Can you work these out from the model? Positions are in its coordinate system, mm. A direction names the side the tool comes from. Round coordinates to 2 decimals unless told otherwise and drop trailing zeros. Order: outer loops, then holes, each group sorted by start corner. A loop starts at its lowest first (then second) coordinate and runs counter-clockwise, first axis right, second up. Notation, with made-up numbers: M 80,-19.5 L 122,-19.5 A23 ccw 122,-10.5 Z; hole C 49.5,33.25 d8. An arc over 180 degrees is marked long. One line per question, with ' | ' between items.
```python
from build123d import *

# Parameters (mm, degrees)
SKETCH_1_W          = 40
SKETCH_1_H          = 40
EXTRUDE_1_DEPTH     = 40
SKETCH_2_R          = 10
CUT_EXTRUDE_1_DEPTH = 41
SKETCH_3_W          = 30
SKETCH_3_H          = 20
CUT_EXTRUDE_2_DEPTH = 20
CUT_EXTRUDE_3_DEPTH = 41
CUT_EXTRUDE_4_DEPTH = 41
SKETCH_7_W          = 10
SKETCH_7_H          = 10
CUT_EXTRUDE_5_DEPTH = 20
CUT_EXTRUDE_6_DEPTH = 21


with BuildPart() as part:
    # 草圖1 → 填料-伸長1 (new body)
    with BuildSketch(Plane(origin=(0, 0, 0), x_dir=(1, 0, 0), z_dir=(0, 1, 0))):
        Rectangle(SKETCH_1_W, SKETCH_1_H)
    extrude(amount=EXTRUDE_1_DEPTH)

    # 草圖2 → 除料-伸長1 (cut, through all)
    with BuildSketch(Plane(origin=(0, 40, 0), x_dir=(1, 0, 0), z_dir=(0, 1, 0))):
        Circle(SKETCH_2_R)
        with BuildLine():
            Line((0, -20), (20, -20))
            Line((20, -20), (20, 0))
            ThreePointArc((20, 0), (14.142135624, -14.142135624), (0, -20))
        make_face()
    extrude(amount=-CUT_EXTRUDE_1_DEPTH, mode=Mode.SUBTRACT)

    # 草圖3 → 除料-伸長2 (cut)
    with BuildSketch(Plane(origin=(20, 0, 0), x_dir=(0, 0, -1), z_dir=(1, 0, 0))):
        with Locations((-5, 30)):
            Rectangle(SKETCH_3_W, SKETCH_3_H)
    extrude(amount=-CUT_EXTRUDE_2_DEPTH, mode=Mode.SUBTRACT)

    # 草圖4 → 除料-伸長3 (cut, through all)
    with BuildSketch(Plane.XY.offset(20)):
        Polygon((20, 30), (10, 30), (10, 20), (0, 20), (0, 30), (-10, 40), (20, 40), align=None)
    extrude(amount=-CUT_EXTRUDE_3_DEPTH, mode=Mode.SUBTRACT)

    # 草圖5 → 除料-伸長4 (cut, through all)
    with BuildSketch(Plane(origin=(20, 0, 0), x_dir=(0, 0, -1), z_dir=(1, 0, 0))):
        Polygon((10, 40), (0, 30), (-10, 30), (-20, 20), (-20, 40), align=None)
    extrude(amount=-CUT_EXTRUDE_4_DEPTH, mode=Mode.SUBTRACT)

    # 草圖7 → 除料-伸長5 (cut)
    with BuildSketch(Plane.XY.offset(20)):
        with Locations((-5, 25)):
            Rectangle(SKETCH_7_W, SKETCH_7_H)
    extrude(amount=-CUT_EXTRUDE_5_DEPTH, mode=Mode.SUBTRACT)

    # 草圖9 → 除料-伸長6 (cut, through all)
    with BuildSketch(Plane(origin=(0, 20, 0), x_dir=(1, 0, 0), z_dir=(0, 1, 0))):
        with BuildLine():
            ThreePointArc((-7.071067812, 7.071067812), (-9.238795325, 3.826834324), (-10, 0))
            Line((-10, 0), (-10, 10))
            Line((-10, 10), (0, 10))
            ThreePointArc((0, 10), (-3.826834324, 9.238795325), (-7.071067812, 7.071067812))
        make_face()
    extrude(amount=CUT_EXTRUDE_6_DEPTH, mode=Mode.SUBTRACT)


solid = part.part
```
(1) Will these pins go through, and if not, where does the flat tip stop? pin 1 Ø24 at (x, z) = (9, 4.5) entering from +Y; pin 2 Ø4 at (x, y) = (-3.5, 22.5) entering from +Z; pin 3 Ø3 at (x, z) = (-15, 2.5) entering from +Y.
Final values:
pin 1: y = 20 | pin 2: z = -10 | pin 3: y = 30
(2) Please list where these lines run through material, in increasing order: probe 1 along X at (y, z) = (6.75, 0); probe 2 along X at (y, z) = (22.5, -15). Write a range as [from, to].
Final values:
probe 1: [-20, -10], [10, 20] | probe 2: [-20, 0], [10, 20]
(3) If we section it at B-B on z = -3.5: Please give me the cut outline in (x, y), plus the area to 3 significant figures.
Final values:
outline: M -20,0 L -9.37,0 L -9.37,20 L -10,20 L -10,33.5 L -20,33.5 Z; M 9.37,0 L 20,0 L 20,20 L 9.37,20 Z | area: 560 mm^2
(4) If we section it at C-C on x = 5.5: Please give me the cut outline in (y, z), plus the area to 3 significant figures.
Final values:
outline: M 0,-20 L 20,-20 L 20,-8.35 L 0,-8.35 Z; M 0,8.35 L 20,8.35 L 20,19.23 L 0,19.23 Z | area: 451 mm^2
(5) If we section it at D-D on z = 16: Please give me the cut outline in (x, y).
Final values:
outline: M -20,0 L 12,0 L 12,20 L -10,20 L -10,24 L -20,24 Z
(6) On a 3-axis mill with a long thin cutter (end or side, diameter ignored), from which of +Z, -Z, +X, -X, +Y, -Y can I reach the whole of each face in a straight line? I mean faces 5 (the flat face through (15, 30, -15)), 6 (the flat face through (-15, 30, 5)), 7 (the flat face through (-5, 28, -10)). Say none if no direction works.
Final values:
face 5: +Z, -Z, +X, +Y | face 6: +Z, +X, -X, +Y | face 7: +Z, +X, +Y
(7) Thinking about a two-plate mould opening in X: for faces 1 (the cylindrical face through (14.297, 10.14, 13.986)), 2 (the flat face through (0, 25, -15)), 3 (the flat face through (10, 25, -15)), 4 (the flat face through (0, 15, -20)), which applies, released by +X, released by -X, zero draft, split by the parting line, or undercut?
Final values:
face 1: released by +X | face 2: undercut | face 3: undercut | face 4: zero draft
(8) If we section it at A-A on y = 23.5: Please give me the cut outline in (x, z).
Final values:
outline: M -20,-20 L 0,-20 L 0,-10 L -10,-10 L -10,16.5 L -20,16.5 Z; M 10,-20 L 20,-20 L 20,-10 L 10,-10 Z
